Part print with two shaded views. Sizes in mm from the minimum x, y, z corner. A direction names the side the tool comes from. Coordinates: 2 decimals unless noted, no trailing zeros. Loops run counter-clockwise (first coordinate to the right, second up) from the corner with the lowest first, then second, coordinate; pieces in that order, holes last. Notation, with made-up numbers: (74, 41.5) -> (103, 41.5) arc R28 cw to (103, 77.5) -> close; hole circle Ø7 at (53.5, -40). An arc over 180 degrees is marked (long way). Answer as a JSON object with one key per item and string values. Group by question number.
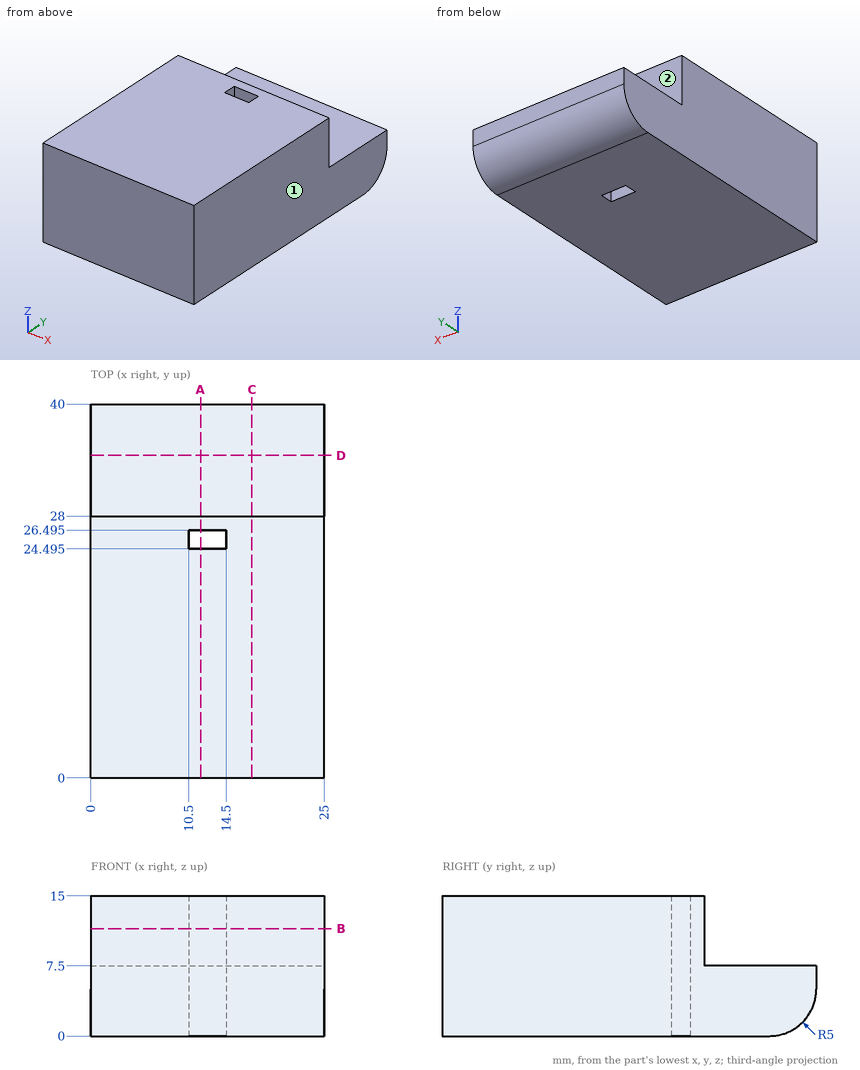
Item 1: Band-saw the part on A-A, the plane x = 11.75. List the corners of the cut face in (y, z) (1 decimal).
Item 2: Band-saw the part on D-D, the plane y = 34.5. List the corners of the cut face in (x, z), and give its area (4 significant figures).
Item 3: Flat gauge pin, fed straight in: P1, Ø8, axis at x = 7.5, z = 12, coming from the +Y side. Where does the tip first touch, or does it go through?
Item 4: Band-saw the part on C-C, the plane x = 17.25. List the corners of the cut face in (y, z).
Item 5: 3-axis set-ups, long thin cutter, end or side, ignore diameter. For the marked faces 1 and 2: which of +Z, -Z, +X, -X, +Y, -Y reach the whole face in a straight line?
Item 6: Band-saw the part on B-B, the plane z = 11.5. List the corners of the cut face in (x, y) (1 decimal), and give its area (3 significant figures).
Item 7: Drill centre lines: L1, parallel to Y at x = 14.25, z = 9.5 (1 decimal); L2, parallel to Y at x = 14, z = 5 (1 decimal); L3, parallel to Y at x = 8, z = 13.5. Where is each one in solid material? Low to high.
Reply:
{
 "1": {"outline": "(0, 0) -> (24.5, 0) -> (24.5, 15) -> (0, 15) -> close; (26.5, 0) -> (35, 0) arc R5 ccw to (40, 5) -> (40, 7.5) -> (28, 7.5) -> (28, 15) -> (26.5, 15) -> close"},
 "2": {"outline": "(0, 0) -> (25, 0) -> (25, 7.5) -> (0, 7.5) -> close", "area": "187.5 mm²"},
 "3": {"P1": "y = 28"},
 "4": {"outline": "(0, 0) -> (35, 0) arc R5 ccw to (40, 5) -> (40, 7.5) -> (28, 7.5) -> (28, 15) -> (0, 15) -> close"},
 "5": {"face 1": "+Z, -Z, +X, +Y, -Y", "face 2": "+Z, +X, -X, +Y"},
 "6": {"outline": "(0, 0) -> (25, 0) -> (25, 28) -> (0, 28) -> close; hole (10.5, 24.5) -> (14.5, 24.5) -> (14.5, 26.5) -> (10.5, 26.5) -> close", "area": "692 mm²"},
 "7": {"L1": "0 to 24.5, 26.5 to 28", "L2": "0 to 24.5, 26.5 to 40", "L3": "0 to 28"}
}
